Read the model definition and answer for the solid it produces. Units are mm, in the model's axes. A direction names the side the tool comes from. Coordinates: 2 decimals unless noted, no trailing zeros. Order: outer loops, then holes, each group sorted by start corner. A loop starts at its lowest first (then second) coordinate and runs counter-clockwise, first axis right, second up. Notation, with made-up numbers: M 12.25,61 L 34.25,61 A6 ccw 34.25,72 Z; hole C 68,8 d2. An arc over 180 degrees is marked long. One line per question, with ' | ' between items. Start each with the question number.
1) Given P1, Ø6, axis at y = 16.5, z = 6.5, coming from the +X side; P2, Ø1, axis at x = -7, z = 22.5, coming from the -Y side; P3, Ø2, axis at x = 25.5, y = 6, coming from the -Z side, each flat-ended and moving along its own axis, determine where each tip first touches the part or whether it passes through.
2) Find section A-A, the plane z = 27.4. Write down the section's boundary in (x, y) (3 decimals), plus the area to 3 significant figures.
3) A tool of negligible diameter and unlimited length cuts with its end or side. For faces 1 (the face through (-4.941, -22.25, 51.257)), 2 (the face through (22.919, -8.494, 19.611)), 3 (the face through (-28, 2, 37)), 4 (the face through (-63.5, -4, 35)), 5 (the face through (-25.126, -1.106, 54.84)), from which of +Z, -Z, +X, -X, +Y, -Y can it reach the whole face along a straight path? Write none if from no direction.
4) The mould has two halves that part along Z. Classify faces 6 (the face through (39.172, -1.707, 35.088)), 7 (the face through (0, 0, 5)), 8 (the face through (0, 0, 0)): +Z half, -Z half, draft (parallel to the pull), parting line (faces both ways), or undercut.
5) Find section C-C, the plane x = 49. Write down the section's boundary in (y, z) (3 decimals), plus the area to 3 significant figures.
6) Find section D-D, the plane z = 49. Write down the section's boundary in (x, y), plus the area to 3 significant figures.
7) Consider probe 1 along Z at (x, y) = (-37, 0) (3 decimals); probe 2 along Z at (x, y) = (26, 0) (3 decimals); probe 3 along Y at (x, z) = (0, 43). Determine where each line is inside the solid, lowest interval first.
8) Find section B-B, the plane x = 0. Write down the section's boundary in (y, z) (3 decimals), plus the area to 3 significant figures.
Autodesk Inventor part; units mm, degrees
ref_plane "YZ Plane" through (0, 0, 0) normal (1, 0, 0) x (0, 1, 0)
ref_plane "XZ Plane" through (0, 0, 0) normal (0, 1, 0) x (-1, 0, 0)
ref_plane "XY Plane" through (0, 0, 0) normal (0, 0, 1) x (1, 0, 0)
sketch "Sketch1" plane through (0, 0, 0) normal (0, 0, 1) x (1, 0, 0)
  circle A0 centre (0, 0) radius 19.05
  dimension "d0" = 38.1
extrude "Extrusion1" add sketch "Sketch1" along normal blind 51.1
sketch "Sketch6" plane through (0, 0, 0) normal (1, 0, 0) x (0, 1, 0)
  line L0 (0, 0) -> (0, 27.4) construction
  circle A0 centre (0, 27.4) radius 9.525
  circle A1 centre (0, 27.4) radius 7.875
  dimension "d22" = 27.4
  dimension "d23" = 19.05
  dimension "d24" = 15.75
extrude "Extrusion6" add sketch "Sketch6" against normal mid plane 127
sketch "Sketch7" plane through (0, 0, 0) normal (1, 0, 0) x (0, 1, 0)
  circle A0 centre (0, 27.4) radius 11.525
  circle A1 centre (0, 27.4) radius 9.525
  dimension "d67" = 2
extrude "Extrusion7" add sketch "Sketch7" along normal mid plane 56
sketch "Sketch13" plane through (0, 0, 51.1) normal (0, 0, 1) x (1, 0, 0)
  circle A0 centre (0, 0) radius 25.15
  circle A1 centre (0, 0) radius 19.05 construction
  dimension "d60" = 50.3
extrude "Extrusion12" add sketch "Sketch13" along normal blind 5
chamfer "Chamfer1" distance 2.515 angle 45 1 edges at (-25.15, 0, 51.1)
sketch "Sketch14" plane through (0, 0, 56.1) normal (0, 0, 1) x (1, 0, 0)
  circle A0 centre (0, 0) radius 17.4
  circle A1 centre (0, 0) radius 19.05 construction
  dimension "d68" = 1.65
extrude "Extrusion13" cut sketch "Sketch14" against normal blind 51.1
sketch "Sketch15" plane through (0, 0, 0) normal (1, 0, 0) x (0, 1, 0)
  circle A0 centre (0, 27.4) radius 7.875
extrude "Extrusion14" cut sketch "Sketch15" along normal through all both and the other way through all
equation "\"d25\" = 2 * d21"
equation "\"d64\" = 0.05 * d60"
equation "\"d69\" = d1"
properties part number "3/4\" DT28" material "Stainless Steel, 316L"
Report:
1) P1: stops at x = 13.44 | P2: stops at y = -17.91 | P3: stops at z = 17.02
2) outline: M -63.5,-9.525 L -28,-9.525 L -28,-11.525 L -15.168,-11.525 A19.05 ccw 15.168,-11.525 L 28,-11.525 L 28,-9.525 L 63.5,-9.525 L 63.5,-7.875 L 15.516,-7.875 A17.4 cw -15.516,-7.875 L -63.5,-7.875 Z; M -63.5,7.875 L -15.516,7.875 A17.4 cw 15.516,7.875 L 63.5,7.875 L 63.5,9.525 L 28,9.525 L 28,11.525 L 15.168,11.525 A19.05 ccw -15.168,11.525 L -28,11.525 L -28,9.525 L -63.5,9.525 Z | area: 540 mm^2
3) face 1: none | face 2: +X | face 3: -X | face 4: +Z, -Z, -X, +Y, -Y | face 5: +Z
4) face 6: undercut | face 7: +Z half | face 8: -Z half
5) outline: C 0,27.4 d19.05; hole C 0,27.4 d15.75 | area: 90.2 mm^2
6) outline: C 0,0 d38.1; hole C 0,0 d34.8 | area: 189 mm^2
7) probe 1: z = 17.875 to 19.525, 35.275 to 36.925 | probe 2: z = 15.875 to 19.525, 35.275 to 38.925 | probe 3: y = -19.05 to -17.4, 17.4 to 19.05
8) outline: M -25.15,53.615 L -22.635,51.1 L -19.05,51.1 L -19.05,0 L 19.05,0 L 19.05,51.1 L 22.635,51.1 L 25.15,53.615 L 25.15,56.1 L 17.4,56.1 L 17.4,5 L -17.4,5 L -17.4,56.1 L -25.15,56.1 Z | area: 414 mm^2
